Check sheet for the modelled part. Datum: model origin and axes. Units: mm. A direction names the side the tool comes from. Coordinates: 2 decimals unless noted, no trailing zeros. Order: outer loops, then holes, each group sorted by start corner. A loop starts at its lowest first (then second) coordinate and runs counter-clockwise, first axis right, second up. Notation, with made-up numbers: (33.5, 78.5) -> (86.5, 78.5) arc R22 ccw to (86.5, 109.5) -> close; hole circle Ø5 at (42.5, 17). An arc over 180 degrees is marked (long way). Put each result on its own line as item: value. Start each with the question number.
```python
from build123d import *

# Parameters (mm, degrees)
F1_DEPTH = 50
F2_W     = 80
F2_H     = 90
F2_W_2   = 3
F2_H_2   = 20
F3_DEPTH = 35
F4_D     = 3
F4_DEPTH = 20
F4_TIP   = 0.9012909285
F5_R     = 5
F6_DEPTH = 10
F7_DEPTH = 15
F8_R     = 3
F9_DEPTH = 60


# Not quite as in the source:
# - a feature names something its author has since deleted; it is built from what else it names


with BuildPart() as f1:
    # F0 (on Front) → F1 (new body, symmetric)
    with BuildSketch(Plane.XZ):
        with BuildLine():
            Line((-59.7125668165, 19.9979344475), (-60.2874331835, 19.9979344475))
            ThreePointArc((-60.2874331835, 19.9979344475), (-79.9994836052, -0.1437203026), (-60, -20))
            ThreePointArc((-60, -20), (-45.8578643763, -14.1421356237), (-40, 0))
            ThreePointArc((-40, 0), (-45.756603922, 14.0401448769), (-59.7125668165, 19.9979344475))
        make_face()
        with BuildLine():
            ThreePointArc((-59.7125668165, 19.9979344475), (-60, 20), (-60.2874331835, 19.9979344475))
            Line((-60.2874331835, 19.9979344475), (-59.7125668165, 19.9979344475))
        make_face()
        with BuildLine():
            ThreePointArc((-40, 0), (-45.8578643763, -14.1421356237), (-60, -20))
            Line((-60, -20), (30, -20))
            ThreePointArc((30, -20), (10.0005163948, -0.1437203026), (29.7125668165, 19.9979344475))
            Line((29.7125668165, 19.9979344475), (-59.7125668165, 19.9979344475))
            ThreePointArc((-59.7125668165, 19.9979344475), (-45.756603922, 14.0401448769), (-40, 0))
        make_face()
        with BuildLine():
            ThreePointArc((29.7125668165, 19.9979344475), (10.0005163948, -0.1437203026), (30, -20))
            ThreePointArc((30, -20), (44.1421356237, -14.1421356237), (50, 0))
            ThreePointArc((50, 0), (44.243396078, 14.0401448769), (30.2874331835, 19.9979344475))
            Line((30.2874331835, 19.9979344475), (29.7125668165, 19.9979344475))
        make_face()
    extrude(amount=F1_DEPTH, both=True)

    # F2 (on face) → F3 (cut)
    with BuildSketch(Plane.XY.offset(19.9979344475)):
        with Locations((-14.7125668165, 0)):
            Rectangle(F2_W, F2_H)
        with Locations((-36.2125668165, 1.5482969955)):
            Rectangle(F2_W_2, F2_H_2, mode=Mode.SUBTRACT)
        Polygon((8.2874331835, 11.3340624973), (8.2874331835, -8.6665749961), (5.1278462474, -8.641347646), (5.2875288045, 11.3580148809), align=None, mode=Mode.SUBTRACT)
    extrude(amount=-F3_DEPTH, mode=Mode.SUBTRACT)

    # F4
    with Locations(Plane.XY.offset(19.9979344475)):
        with Locations((-57.2125668165, 47.5), (27.7874331835, 47.5), (27.7874331835, -47.5), (-57.2125668165, -47.5)):
            Hole(F4_D / 2, depth=F4_DEPTH)
            with Locations((0, 0, -(F4_DEPTH + F4_TIP / 2))):  # 118° drill point
                Cone(0, F4_D / 2, F4_TIP, mode=Mode.SUBTRACT)

    # F5 (on face) → F6 (cut)
    with BuildSketch(Plane(origin=(0, 50, 0), x_dir=(-1, 0, 0), z_dir=(0, 1, 0))):
        with Locations((-12.6515543088, 0)):
            Circle(F5_R)
    extrude(amount=-F6_DEPTH, mode=Mode.SUBTRACT)

    # F7 (add): faces of the model
    f7_faces = [f1.faces().sort_by_distance(p)[0] for p in [
        (-36.2125668165, 1.5482969955, 19.9979344475),
        (6.7472153787, 1.2596232378, 19.9979344475),
    ]]
    extrude(f7_faces, amount=F7_DEPTH)

    # F8 (on face) → F9 (cut)
    with BuildSketch(Plane(origin=(-37.7125668165, 0, 0), x_dir=(0, -1, 0), z_dir=(-1, 0, 0))):
        with Locations((-1.5482969955, 29.857664355)):
            Circle(F8_R)
    extrude(amount=-F9_DEPTH, mode=Mode.SUBTRACT)


solid = f1.part
```
1) Scan lines: line 1 along Y through (x, z) = (-35, -5.5); line 2 along Y through (x, z) = (-57, 7.5); line 3 along Y through (x, z) = (15, -6). Record each from-to range of solid material in increasing order. Write a range as [from, to].
2) Access from +Z, -Z, +X, -X, +Y, -Y to the whole of each face (thin tool, end or side, straight path). Record for faces 1 (the flat face through (-16, -50, 0)), 2 (the cylindrical face through (-56.887, -48.964, 9.858)).
3) Sectioned sample at A-A (z = 11). Record the boundary of the cut face in (x, y), plus the area to 3 significant figures.
4) Gauge pin test, flat ends, axial feed: pin 1 (1 mm diameter, centred on x = -11, y = 37.5, fed in from +Z); pin 2 (2.5 mm diameter, centred on x = -57.21, y = -47.5, fed in from +Z); pin 3 (9.5 mm diameter, centred on y = 1.55, z = 29.86, fed in from -X). Record the tip position at first contact, or that the pin passes through.
5) Sectioned sample at B-B (y = -35.5). Record the boundary of the cut face in (x, z).
6) Mould release check, pull along Z, two halves, no side actions. Record for faces 3 (the flat face through (25.5, 3.5, 19.998)), 4 (the cylindrical face through (49.99, -0.7, -0.58)), 5 (the flat face through (-36, 11.548, 10)), 6 (the cylindrical face through (6.71, 2.2, 26.93)): +Z half, -Z half, draft (parallel to the pull), parting line (faces both ways), or undercut.
7) Sectioned sample at C-C (x = -51). Record the boundary of the cut face in (y, z), plus the area to 3 significant figures.
8) Sectioned sample at D-D (z = -13). Record the boundary of the cut face in (x, y).
Entries:
1. line 1: y = [-50, -45], [-8.45, 11.55], [45, 50]
1. line 2: y = [-50, -48.98], [-46.02, 46.02], [48.98, 50]
1. line 3: y = [-50, -45], [45, 50]
2. face 1: +Z, -Z, +X, -X, -Y
2. face 2: +Z
3. outline: (-76.7, -50) -> (46.7, -50) -> (46.7, 50) -> (-76.7, 50) -> close; (-37.71, -8.45) -> (-34.71, -8.45) -> (-34.71, 11.55) -> (-37.71, 11.55) -> close; (5.13, -8.64) -> (8.29, -8.67) -> (8.29, 11.33) -> (5.29, 11.36) -> close; hole circle Ø3 at (-57.21, -47.5); hole circle Ø3 at (-57.21, 47.5); hole (-54.71, -45) -> (25.29, -45) -> (25.29, 45) -> (-54.71, 45) -> close; hole circle Ø3 at (27.79, -47.5); hole circle Ø3 at (27.79, 47.5)
3. area: 5,230 mm2
4. pin 1: stops at z = -15
4. pin 2: stops at z = -0.15
4. pin 3: stops at x = -37.71
5. outline: (-60, -20) -> (30, -20) arc R20 ccw to (30.29, 20) -> (25.29, 20) -> (25.29, -15) -> (-54.71, -15) -> (-54.71, 20) -> (-59.71, 20) arc R20 ccw (long way) to start
6. face 3: +Z half
6. face 4: parting line
6. face 5: draft
6. face 6: undercut
7. outline: (-50, -20) -> (50, -20) -> (50, 20) -> (45, 20) -> (45, -15) -> (-45, -15) -> (-45, 20) -> (-50, 20) -> close
7. area: 850 mm2
8. outline: (-75.2, -50) -> (45.2, -50) -> (45.2, 50) -> (-75.2, 50) -> close; (-37.71, -8.45) -> (-34.71, -8.45) -> (-34.71, 11.55) -> (-37.71, 11.55) -> close; (5.13, -8.64) -> (8.29, -8.67) -> (8.29, 11.33) -> (5.29, 11.36) -> close; hole (-54.71, -45) -> (25.29, -45) -> (25.29, 45) -> (-54.71, 45) -> close
